```python
from build123d import *

# Parameters (mm, degrees)
F0_R     = 3
F1_DEPTH = 20
F3_DEPTH = 5
F4_SIZE  = 0.5
F5_DEPTH = 56.5


with BuildPart() as f1:
    # F0 (on Top) → F1 (new body)
    with BuildSketch(Plane.XY):
        Circle(F0_R)
    extrude(amount=F1_DEPTH)

    # F2 (on face) → F3 (join)
    with BuildSketch(Plane.XY.offset(20)):
        Polygon((0, -5.7735026919), (5, -2.8867513459), (5, 2.8867513459), (0, 5.7735026919), (-5, 2.8867513459), (-5, -2.8867513459), align=None)
    extrude(amount=F3_DEPTH)

    # F4
    f4_edges = [f1.edges().sort_by_distance(p)[0] for p in [
        (-2.5, -4.330127, 25),
        (2.5, -4.330127, 25),
        (5, 0, 25),
        (2.5, 4.330127, 25),
        (-2.5, 4.330127, 25),
        (-5, 0, 25),
        (-2.5, -4.330127, 20),
        (-5, 0, 20),
        (2.5, -4.330127, 20),
        (-2.5, 4.330127, 20),
        (5, 0, 20),
        (2.5, 4.330127, 20),
        (-3, 0, 20),
    ]]
    chamfer(f4_edges, length=F4_SIZE)

    # F5 (add): a face of the model
    f5_faces = [f1.faces().sort_by_distance(p)[0] for p in [
        (0, 0, 0),
    ]]
    extrude(f5_faces, amount=F5_DEPTH)


solid = f1.part
```
Verification items for the finished model (mm, model axes). A direction names the side the tool comes from. Coordinates: 2 decimals unless noted, no trailing zeros. Order: outer loops, then holes, each group sorted by start corner. A loop starts at its lowest first (then second) coordinate and runs counter-clockwise, first axis right, second up. Notation, with made-up numbers: (18.5, -19) -> (43.5, -19) arc R29 ccw to (43.5, 12) -> close; hole circle Ø4 at (-7.75, -1.75). An arc over 180 degrees is marked (long way). Put each result on its own line as item: value. Start each with the question number.
1) Tool access check on faces 1 (the flat face through (5, 0, 22)), 2 (the cylindrical face through (-3, 0, -18)). Record the directions out of +Z, -Z, +X, -X, +Y, -Y that give a thin tool (end or side, any length) a straight path to the whole face; none if there is none.
2) Material ranges on L1, parallel to Y at x = 0, z = -2; L2, parallel to Z at x = 3.5, y = 0.5; L3, parallel to X at y = 2.5, z = -17.5, recorded low to high.
3) Cross-section at B-B (z = -39). Enter the section's corners in (x, y), plus the area to 3 significant figures.
4) Cross-section at A-A (y = 0). Enter the section's corners in (x, z), plus the area to 3 significant figures.
5) Go/stop test with flat-tipped pins: pin 1 (3 mm diameter, centred on y = -4, z = -27.5, fed in from +X); pin 2 (6 mm diameter, centred on y = 3, z = 3.5, fed in from +X); pin 3 (3 mm diameter, centred on x = 0.5, z = -45.5, fed in from +Y). Record where each tip stops, or that it passes through.
Geometry check:
1. face 1: +Z, -Z, +X, +Y, -Y
1. face 2: -Z
2. L1: y = -3 to 3
2. L2: z = 20 to 25
2. L3: x = -1.66 to 1.66
3. outline: circle Ø6 at (0, 0)
3. area: 28.3 mm^2
4. outline: (-5, 20.5) -> (-4.5, 20) -> (-3.5, 20) -> (-3, 19.5) -> (-3, -56.5) -> (3, -56.5) -> (3, 19.5) -> (3.5, 20) -> (4.5, 20) -> (5, 20.5) -> (5, 24.5) -> (4.5, 25) -> (-4.5, 25) -> (-5, 24.5) -> close
4. area: 509 mm^2
5. pin 1: stops at x = 1.66
5. pin 2: stops at x = 3
5. pin 3: stops at y = 3
